Can you work these out from the model? Positions are in its coordinate system, mm. Face numbers are marked on the shaded views. A direction names the side the tool comes from. Give positions to 0.01 mm unless a question says otherwise; leave off trailing zeros. Loops run counter-clockwise (first coordinate to the right, second up) from the corner with the lowest first, then second, coordinate; pieces in that order, holes last. Notation, with made-up numbers: (14.5, -34) - (33.5, -34) arc R10 ccw to (33.5, -27) - close; hole circle Ø5 at (-22, 77). An arc over 180 degrees is marked (long way). Answer in a Markdown table with one row per item.
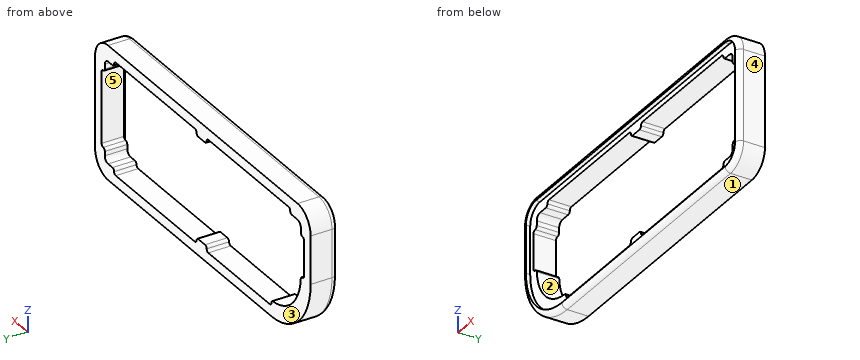
from build123d import *

# Parameters (mm, degrees)
F2_DEPTH = 25
F3_R     = 5
F4_DEPTH = 4
F6_DEPTH = 25


with BuildPart() as f2:
    # F1 (on Front) → F2 (new body)
    with BuildSketch(Plane.XZ):
        with BuildLine():
            Line((-4.9999973178, 100), (-4.9999973178, 55))
            ThreePointArc((-4.9999973178, 55), (12.5735950254, 12.5735950254), (55, -4.9999973178))
            Line((55, -4.9999973178), (305, -4.9999973178))
            ThreePointArc((305, -4.9999973178), (319.1421337271, 0.8578662729), (324.9999973178, 15))
            Line((324.9999973178, 15), (324.9999973178, 100))
            ThreePointArc((324.9999973178, 100), (319.1421337271, 114.1421337271), (305, 119.9999973178))
            Line((305, 119.9999973178), (15, 119.9999973178))
            ThreePointArc((15, 119.9999973178), (0.8578662729, 114.1421337271), (-4.9999973178, 100))
        make_face()
    extrude(amount=F2_DEPTH)

    # F3
    f3_edges = [f2.edges().sort_by_distance(p)[0] for p in [
        (160, -25, 119.999997),
        (0.857866, -25, 114.142134),
        (-4.999997, -25, 77.5),
        (12.573595, -25, 12.573595),
        (180, -25, -4.999997),
        (319.142134, -25, 0.857866),
        (324.999997, -25, 57.5),
        (319.142134, -25, 114.142134),
    ]]
    fillet(f3_edges, radius=F3_R)

    # F2_face (on face) + F0 (on Front) + F2_face1 (on face) → F4 (cut)
    with BuildSketch(Plane(origin=(162.4531537348, -25, 58.2425840515), x_dir=(1, 0, 0), z_dir=(0, -1, 0))):
        with BuildLine():
            Line((142.5468462652, 56.7574132663), (-147.4531537348, 56.7574132663))
            ThreePointArc((-147.4531537348, 56.7574132663), (-158.059753556, 52.3640157697), (-162.4531510526, 41.7574159485))
            Line((-162.4531510526, 41.7574159485), (-162.4531510526, -3.2425840515))
            ThreePointArc((-162.4531510526, -3.2425840515), (-146.3440248034, -42.1334551202), (-107.4531537348, -58.2425813693))
            Line((-107.4531537348, -58.2425813693), (142.5468462652, -58.2425813693))
            ThreePointArc((142.5468462652, -58.2425813693), (153.1534460864, -53.8491838727), (157.546843583, -43.2425840515))
            Line((157.546843583, -43.2425840515), (157.546843583, 41.7574159485))
            ThreePointArc((157.546843583, 41.7574159485), (153.1534460864, 52.3640157697), (142.5468462652, 56.7574132663))
        make_face()
    with BuildSketch(Plane.XZ):
        with BuildLine():
            Line((186.9708299637, 115), (189.8719519377, 0))
            Line((189.8719519377, 0), (305, 0))
            ThreePointArc((305, 0), (315.6066017178, 4.3933982822), (320, 15))
            Line((320, 15), (320, 100))
            ThreePointArc((320, 100), (315.6066017178, 110.6066017178), (305, 115))
            Line((305, 115), (186.9708299637, 115))
        make_face()
    with BuildSketch(Plane(origin=(162.5693555517, 0, 58.3192422461), x_dir=(1, 0, 0), z_dir=(0, 1, 0))):
        with BuildLine():
            Line((-167.5693528695, 3.3192422461), (-167.5693528695, -41.6807577539))
            ThreePointArc((-167.5693528695, -41.6807577539), (-161.7114892788, -55.8228914811), (-147.5693555517, -61.6807550717))
            Line((-147.5693555517, -61.6807550717), (142.4306444483, -61.6807550717))
            ThreePointArc((142.4306444483, -61.6807550717), (156.5727781754, -55.8228914811), (162.4306417661, -41.6807577539))
            Line((162.4306417661, -41.6807577539), (162.4306417661, 43.3192422461))
            ThreePointArc((162.4306417661, 43.3192422461), (156.5727781754, 57.4613759732), (142.4306444483, 63.3192395638))
            Line((142.4306444483, 63.3192395638), (-107.5693555517, 63.3192395638))
            ThreePointArc((-107.5693555517, 63.3192395638), (-149.9957605263, 45.7456472206), (-167.5693528695, 3.3192422461))
        make_face()
    extrude(amount=-F4_DEPTH, dir=(0, -1, 0), mode=Mode.SUBTRACT)

    # F5 (on face) → F6 (cut)
    with BuildSketch(Plane.XZ.offset(21)):
        with BuildLine():
            Line((298.2851588726, 10.0000026822), (305, 10.0000026822))
            ThreePointArc((305, 10.0000026822), (308.5355320093, 11.4644679907), (309.9999973178, 15))
            Line((309.9999973178, 15), (309.9999973178, 19.0326044708))
            ThreePointArc((309.9999973178, 19.0326044708), (310.7322303648, 20.8003714238), (312.4999973178, 21.5326044708))
            ThreePointArc((312.4999973178, 21.5326044708), (314.2677642708, 22.2648375179), (314.9999973178, 24.0326044708))
            Line((314.9999973178, 24.0326044708), (314.9999973178, 90.5494615436))
            ThreePointArc((314.9999973178, 90.5494615436), (314.2677642708, 92.3172284965), (312.4999973178, 93.0494615436))
            ThreePointArc((312.4999973178, 93.0494615436), (310.7322303648, 93.7816945906), (309.9999973178, 95.5494615436))
            Line((309.9999973178, 95.5494615436), (309.9999973178, 100))
            ThreePointArc((309.9999973178, 100), (308.5355320093, 103.5355320093), (305, 104.9999973178))
            Line((305, 104.9999973178), (298.2851588726, 104.9999973178))
            ThreePointArc((298.2851588726, 104.9999973178), (296.5173919196, 105.7322303648), (295.7851588726, 107.4999973178))
            ThreePointArc((295.7851588726, 107.4999973178), (295.0529258256, 109.2677642708), (293.2851588726, 109.9999973178))
            Line((293.2851588726, 109.9999973178), (172.0636063814, 109.9999973178))
            ThreePointArc((172.0636063814, 109.9999973178), (170.2958394284, 109.2677642708), (169.5636063814, 107.4999973178))
            ThreePointArc((169.5636063814, 107.4999973178), (168.8313733344, 105.7322303648), (167.0636063814, 104.9999973178))
            Line((167.0636063814, 104.9999973178), (156.6095525026, 104.9999973178))
            ThreePointArc((156.6095525026, 104.9999973178), (154.8417855497, 105.7322303648), (154.1095525026, 107.4999973178))
            ThreePointArc((154.1095525026, 107.4999973178), (153.3773194556, 109.2677642708), (151.6095525026, 109.9999973178))
            Line((151.6095525026, 109.9999973178), (28.7736566365, 109.9999973178))
            ThreePointArc((28.7736566365, 109.9999973178), (27.0058896835, 109.2677642708), (26.2736566365, 107.4999973178))
            ThreePointArc((26.2736566365, 107.4999973178), (25.5414235894, 105.7322303648), (23.7736566365, 104.9999973178))
            Line((23.7736566365, 104.9999973178), (15, 104.9999973178))
            ThreePointArc((15, 104.9999973178), (11.4644679907, 103.5355320093), (10.0000026822, 100))
            Line((10.0000026822, 100), (10.0000026822, 95.5494615436))
            ThreePointArc((10.0000026822, 95.5494615436), (9.2677696352, 93.7816945906), (7.5000026822, 93.0494615436))
            ThreePointArc((7.5000026822, 93.0494615436), (5.7322357292, 92.3172284965), (5.0000026822, 90.5494615436))
            Line((5.0000026822, 90.5494615436), (5.0000026822, 57.5))
            ThreePointArc((5.0000026822, 57.5), (5.7322357292, 55.732233047), (7.5000026822, 55))
            Line((7.5000026822, 55), (7.5658377834, 55))
            ThreePointArc((7.5658377834, 55), (9.2864557847, 54.3136906278), (10.0623727779, 52.6315789548))
            ThreePointArc((10.0623727779, 52.6315789548), (23.1801967432, 23.1801967432), (52.6315789548, 10.0623727779))
            ThreePointArc((52.6315789548, 10.0623727779), (54.3136906278, 9.2864557847), (55, 7.5658377834))
            Line((55, 7.5658377834), (55, 7.5000026822))
            ThreePointArc((55, 7.5000026822), (55.732233047, 5.7322357292), (57.5, 5.0000026822))
            Line((57.5, 5.0000026822), (151.6095525026, 5.0000026822))
            ThreePointArc((151.6095525026, 5.0000026822), (153.3773194556, 5.7322357292), (154.1095525026, 7.5000026822))
            ThreePointArc((154.1095525026, 7.5000026822), (154.8417855497, 9.2677696352), (156.6095525026, 10.0000026822))
            Line((156.6095525026, 10.0000026822), (167.0636063814, 10.0000026822))
            ThreePointArc((167.0636063814, 10.0000026822), (168.8313733344, 9.2677696352), (169.5636063814, 7.5000026822))
            ThreePointArc((169.5636063814, 7.5000026822), (170.2958394284, 5.7322357292), (172.0636063814, 5.0000026822))
            Line((172.0636063814, 5.0000026822), (293.2851588726, 5.0000026822))
            ThreePointArc((293.2851588726, 5.0000026822), (295.0529258256, 5.7322357292), (295.7851588726, 7.5000026822))
            ThreePointArc((295.7851588726, 7.5000026822), (296.5173919196, 9.2677696352), (298.2851588726, 10.0000026822))
        make_face()
    extrude(amount=-F6_DEPTH, mode=Mode.SUBTRACT)


solid = f2.part
Q1. If we mould it in two halves opening along X, with no side actions, what happens to the marked faces 3, 4 and 5? For each: released by +X, released by -X, zero draft, split by the parting line, or undercut.
Checked values:
| item | result |
|---|---|
| face 3 | zero draft |
| face 4 | released by +X |
| face 5 | undercut |
Q2. If I drill on line 1 (Z direction, x = 53, y = -8.25); line 2 (Z direction, x = 253, y = -14.5); line 3 (X direction, y = -3.25, z = 79), over which ranges is the centre line in solid material (lowest first)? Write a range as [from, to].
Checked values:
| item | result |
|---|---|
| line 1 | z = [-4.97, 10.02], [110, 120] |
| line 2 | z = [-5, 5], [110, 120] |
| line 3 | x = [-5, 5], [315, 325] |
Q3. For pin 1 (12 mm diameter, centred on y = -10.5, z = 39, fed in from -X); pin 2 (2.5 mm diameter, centred on x = 18.5, y = -12, fed in from -Z); pin 3 (12 mm diameter, centred on x = 54.5, z = 20.5, fed in from -Y); pin 4 (2 mm diameter, centred on y = -23, z = 73.5, fed in from +X), each with a flat end and sliding along its axis, tell me the tip position at first contact or that it passes through.
Checked values:
| item | result |
|---|---|
| pin 1 | stops at x = -4.16 |
| pin 2 | stops at z = 6.45 |
| pin 3 | passes through |
| pin 4 | stops at x = 324.58 |
Q4. Imagine slicing it at A-A, the plane x = 128.5. Write out the boundary of the cut face in (y, z), and give its area (3 significant figures).
Checked values:
| item | result |
|---|---|
| outline | (-25, 0) arc R5 ccw to (-20, -5) - (0, -5) - (0, 5) - (-21, 5) - (-21, 0) - close; (-25, 115) - (-21, 115) - (-21, 110) - (0, 110) - (0, 120) - (-20, 120) arc R5 ccw to start |
| area | 449 mm² |
Q5. On a 3-axis mill with a long thin cutter (end or side, diameter ignored), from which of +Z, -Z, +X, -X, +Y, -Y can I reach the whole of each face in a straight line? I mean the marked faces 1 and 2. Say none if no direction works.
Checked values:
| item | result |
|---|---|
| face 1 | -Z, +X, -X, +Y, -Y |
| face 2 | +Y, -Y |
